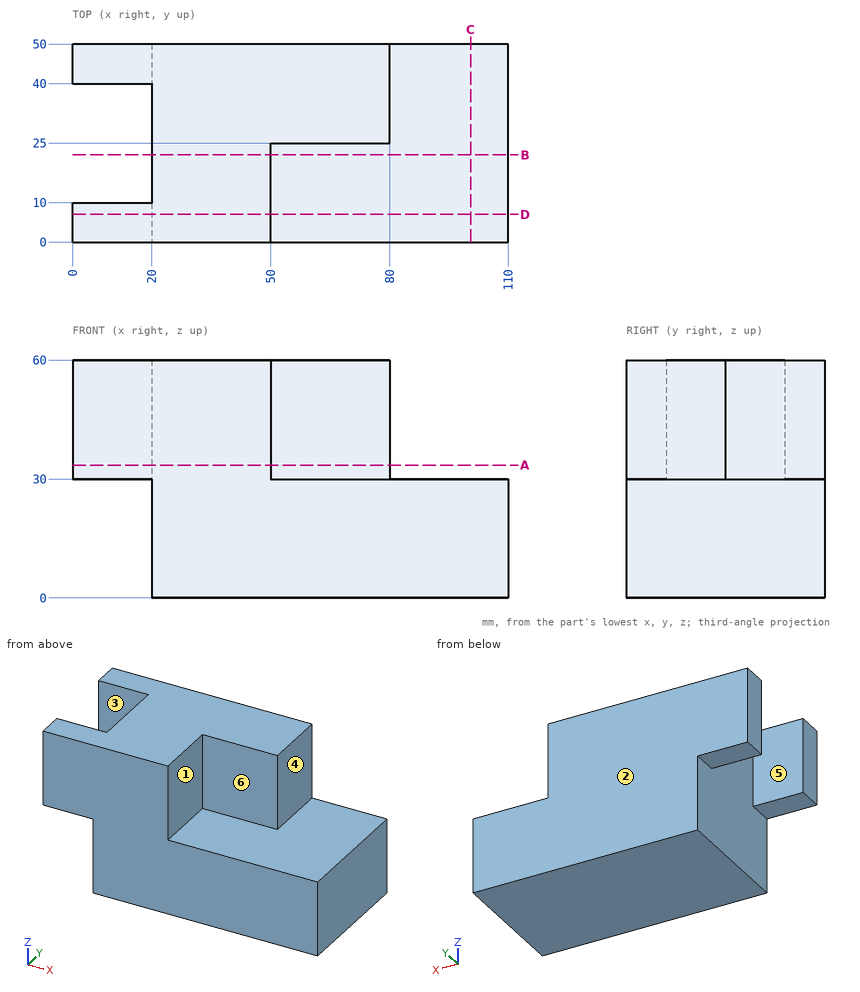
For this review, use the dimensioned drawing (mm, ordinates from the lowest corner) and the shaded views. A direction names the side the tool comes from. Round coordinates to 2 decimals unless told otherwise and drop trailing zeros. Write each loop counter-clockwise with the first axis right and the second up, starting at its lowest first coordinate (ties: lowest second). Pieces come first, ordered by that corner, then holes. Notation, with made-up numbers: (82, 27.5) -> (102, 27.5) arc R12 ccw to (102, 44.5) -> close; hole circle Ø5 at (-32.5, 64.5). An arc over 180 degrees is marked (long way). Use one line per item in the form item = value.
Q1. Machinability: for the marked faces 4, 5 and 6, which of the approach directions +Z, -Z, +X, -X, +Y, -Y give a long, thin tool a straight path to every point of the face, cutting with its end or side? Answer none if there is none.
Resolved:
face_4 = +Z, +X, +Y, -Y
face_5 = +Z, -Z, -X
face_6 = +Z, +X, -Y
Q2. Consider section C-C (x = 100.5). State the section outline as (y, z) points.
Resolved:
outline = (0, 0) -> (50, 0) -> (50, 30) -> (0, 30) -> close
Q3. Clearance check with flat-ended pins moving along their axes: pin 1 Ø2 at (y, z) = (42, 52) entering from +X; pin 2 Ø5 at (x, y) = (6, 47) entering from -Z; pin 3 Ø10 at (x, z) = (71.5, 53.5) entering from -Y. State where each tip first meets the part, or that it passes through.
Resolved:
pin_1 = 80
pin_2 = 30
pin_3 = 25
Q4. Consider section D-D (y = 7). State the section outline as (x, z) points.
Resolved:
outline = (0, 30) -> (20, 30) -> (20, 0) -> (110, 0) -> (110, 30) -> (50, 30) -> (50, 60) -> (0, 60) -> close
Q5. The part is to be moulded in two halves that separate along Y. For the marked faces 1, 2 and 3, say which applies: released by +Y, released by -Y, zero draft, split by the parting line, or undercut.
Resolved:
face_1 = zero draft
face_2 = released by +Y
face_3 = undercut
Q6. Consider section B-B (y = 22). State the section outline as (x, z) points.
Resolved:
outline = (20, 0) -> (110, 0) -> (110, 30) -> (50, 30) -> (50, 60) -> (20, 60) -> close
Q7. To check wall thickness, follow probe 1 along X at (y, z) = (9.5, 55.5); probe 2 along X at (y, z) = (28.5, 3); probe 3 along Y at (x, z) = (59.5, 44). State the ranges of each line that lie inside material, in increasing order. Write a range as from..to.
Resolved:
probe_1 = 0..50
probe_2 = 20..110
probe_3 = 25..50
Q8. Consider section A-A (z = 33.5). State the section outline as (x, y) points, then the cut area to 3 significant figures.
Resolved:
outline = (0, 0) -> (50, 0) -> (50, 25) -> (80, 25) -> (80, 50) -> (0, 50) -> (0, 40) -> (20, 40) -> (20, 10) -> (0, 10) -> close
area = 2,650 mm²
